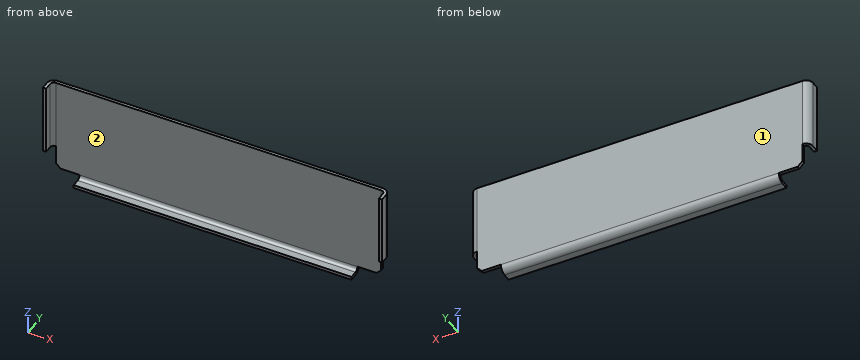
from build123d import *

# Parameters (mm, degrees)
F1_DEPTH = 101.6
F2_W     = 347.66504
F2_H     = 7.38632
F3_DEPTH = 3.41884
F4_W     = 347.66504
F4_H     = 3.41884
F5_DEPTH = 11.90498
F6_R     = 3.96748
F7_R     = 7.38632
F8_W     = 7.38632
F8_H     = 25.4
F8_W_2   = 25.4
F8_H_2   = 7.38632
F9_DEPTH = 15.32382
F10_SIZE = 5.08


# Not quite as in the source:
# - a feature names something its author has since deleted; it is built from what else it names


with BuildPart() as f1:
    # F0 (on Top) → F1 (new body)
    with BuildSketch(Plane.XY):
        Polygon((-3.41884, 0), (0, 0), (0, 11.90498), (355.6, 11.90498), (355.6, 0), (359.01884, 0), (359.01884, 15.32382), (-3.41884, 15.32382), align=None)
    extrude(amount=F1_DEPTH)

    # F2 (on face) → F3 (join, through all)
    with BuildSketch(Plane(origin=(0, 15.32382, 0), x_dir=(-1, 0, 0), z_dir=(0, 1, 0))):
        with Locations((-177.8, -3.69316)):
            Rectangle(F2_W, F2_H)
    extrude(amount=-F3_DEPTH)

    # F4 (on face) → F5 (join, through all)
    with BuildSketch(Plane.XZ.offset(-11.90498)):
        with Locations((177.8, -5.6769)):
            Rectangle(F4_W, F4_H)
    extrude(amount=F5_DEPTH)

    # F6
    f6_edges = [f1.edges().sort_by_distance(p)[0] for p in [
        (0, 11.90498, 50.8),
        (355.6, 11.90498, 50.8),
        (177.8, 11.90498, -3.96748),
    ]]
    fillet(f6_edges, radius=F6_R)

    # F7
    f7_edges = [f1.edges().sort_by_distance(p)[0] for p in [
        (-3.41884, 15.32382, 50.8),
        (359.01884, 15.32382, 50.8),
        (177.8, 15.32382, -7.38632),
    ]]
    fillet(f7_edges, radius=F7_R)

    # F8 (on face) → F9 (cut, through all)
    with BuildSketch(Plane(origin=(0, 15.32382, 0), x_dir=(-1, 0, 0), z_dir=(0, 1, 0))):
        with Locations((-355.32568, 12.7)):
            Rectangle(F8_W, F8_H)
        with Locations((-338.93252, -3.69316)):
            Rectangle(F8_W_2, F8_H_2)
        with Locations((-0.27432, 12.7)):
            Rectangle(F8_W, F8_H)
        with Locations((-16.66748, -3.69316)):
            Rectangle(F8_W_2, F8_H_2)
    extrude(amount=-F9_DEPTH, mode=Mode.SUBTRACT)

    # F10
    f10_edges = [f1.edges().sort_by_distance(p)[0] for p in [
        (351.63252, 13.6144, 0),
        (3.96748, 13.6144, 0),
    ]]
    chamfer(f10_edges, length=F10_SIZE)


solid = f1.part
Could you check a few things on this model? Use its own coordinates, in mm. Face numbers are marked on the shaded views. A direction names the side the tool comes from. Coordinates: 2 decimals unless noted, no trailing zeros. Write each loop counter-clockwise with the first axis right and the second up, starting at its lowest first coordinate (ties: lowest second). Pieces come first, ordered by that corner, then holes. Notation, with made-up numbers: (81, 42.25) - (102, 42.25) arc R14 cw to (102, 50.25) - close; hole circle Ø4 at (62.5, 37). An arc over 180 degrees is marked (long way). Put each result on its own line as item: value. Start each with the question number.
Q1. Which directions (+Z, -Z, +X, -X, +Y, -Y) give clear straight access to the entire face, cutting with the end or side of a thin tool? Please do the marked faces 1 and 2.
Q2. I want a section at A-A on y = 2.5. Write out the boundary of the cut face in (x, z).
Q3. I'm going to push flat-ended pins straight in: P1, Ø1.7, axis at x = 331.5, y = 14, coming from the -Z side; P2, Ø6, axis at y = 8, z = -5, coming from the +X side; P3, Ø1, axis at x = 209.5, z = 47, coming from the -Y side (3 decimals); P4, Ø2, axis at x = 353.5, y = 6, coming from the -Z side. Where does each tip first touch, or does it pass through?
Q4. I want a section at C-C on x = 249. Write out the boundary of the cut face in (y, z), plus the area to 3 significant figures.
Q5. Please list where these lines run through material, in increasing order: L1, parallel to X at y = 8.5, z = 72; L2, parallel to Y at x = 327.5, z = 34; L3, parallel to Z at x = 86.5, y = 4.75.
Q6. I want a section at B-B on z = 50. Write out the boundary of the cut face in (x, y).
Q7. I want a section at D-D on z = 12.5. Write out the boundary of the cut face in (x, y).
Checks:
1. face 1: +Z, -Z, +X, -X, +Y
1. face 2: +Z, -Y
2. outline: (-3.42, 25.4) - (0, 25.4) - (0, 101.6) - (-3.42, 101.6) - close; (29.37, -7.39) - (326.23, -7.39) - (326.23, -3.97) - (29.37, -3.97) - close; (355.6, 25.4) - (359.02, 25.4) - (359.02, 101.6) - (355.6, 101.6) - close
3. P1: z = 0
3. P2: x = 326.23
3. P3: y = 11.905
3. P4: through
4. outline: (0, -7.39) - (7.94, -7.39) arc R7.39 ccw to (15.32, 0) - (15.32, 101.6) - (11.9, 101.6) - (11.9, 0) arc R3.97 cw to (7.94, -3.97) - (0, -3.97) - close
4. area: 405 mm²
5. L1: -3.4 to 0.04, 355.56 to 359
5. L2: 11.9 to 15.32
5. L3: -7.39 to -3.97
6. outline: (-3.42, 0) - (0, 0) - (0, 7.94) arc R3.97 cw to (3.97, 11.9) - (351.63, 11.9) arc R3.97 cw to (355.6, 7.94) - (355.6, 0) - (359.02, 0) - (359.02, 7.94) arc R7.39 ccw to (351.63, 15.32) - (3.97, 15.32) arc R7.39 ccw to (-3.42, 7.94) - close
7. outline: (3.97, 11.9) - (351.63, 11.9) - (351.63, 15.32) - (3.97, 15.32) - close
